```python
from build123d import *

# Parameters (mm, degrees)
F0_R         = 150.3237387913
F0_R_2       = 73.6926609148
F1_DEPTH     = 254
F2_R         = 20.32
F3_R         = 112.9256404591
F3_R_2       = 87.0757104376
F4_DEPTH     = 25.4
F5_R         = 128.6901964601
F6_DEPTH     = 63.5
F7_T4_DEPTH  = 60.7095224794
F7_S5_R      = 128.6901964601
F7_T6_DEPTH  = 32
F7_T10_DEPTH = 60.7095224794
F7_S11_R     = 128.6901964601
F7_T12_DEPTH = 32
F7_T16_DEPTH = 60.7095224794
F7_S17_R     = 128.6901964601
F7_T18_DEPTH = 32
F7_T22_DEPTH = 60.7095224794
F7_S23_R     = 128.6901964601
F7_T24_DEPTH = 32


# Not quite as in the source:
# - a fillet or chamfer that OpenCascade refuses, or shapes differently, is made with other operations: its cross-section is extruded or revolved along the edge and cut away or added


with BuildPart() as f1:
    # F0 (on Front) → F1 (new body)
    with BuildSketch(Plane.XZ):
        Circle(F0_R)
        Circle(F0_R_2, mode=Mode.SUBTRACT)
    extrude(amount=F1_DEPTH)

    # F2
    f2_edges = [f1.edges().sort_by_distance(p)[0] for p in [
        (-150.323739, -254, 0),
    ]]
    fillet(f2_edges, radius=F2_R)

    # F3 (on face) → F4 (join)
    with BuildSketch(Plane(origin=(0, 0, 0), x_dir=(-1, 0, 0), z_dir=(0, 1, 0))):
        Circle(F3_R)
        Circle(F3_R_2, mode=Mode.SUBTRACT)
    extrude(amount=F4_DEPTH)

    # F5 (on Top) → F6 (join, symmetric)
    with BuildSketch(Plane.XY):
        Circle(F5_R)
    extrude(amount=F6_DEPTH, both=True)

    # F7: fillet of radius 5.08 on 4 edges, made by hand


with BuildPart() as f7_tool2:
    # F7_s3 → F7_t4 (new body)
    with BuildSketch(Plane.YZ.offset(-80.6806739807)):
        with BuildLine():
            ThreePointArc((0, -68.58), (1.4878975516, -64.9878975516), (5.08, -63.5))
            Line((5.08, -63.5), (0, -63.5))
            Line((0, -63.5), (0, -68.58))
        make_face()
    extrude(amount=-F7_T4_DEPTH)

    # F7_s5 → F7_t6 (intersect, symmetric)
    with BuildSketch(Plane.XY.offset(-66)):
        Circle(F7_S5_R)
    extrude(amount=F7_T6_DEPTH, both=True, mode=Mode.INTERSECT)


with BuildPart() as f1_1:
    add(f1.part)

    # F7_t1: union F7_tool2
    add(f7_tool2.part)


with BuildPart() as f7_tool8:
    # F7_s9 → F7_t10 (new body)
    with BuildSketch(Plane.YZ.offset(141.3901964601)):
        with BuildLine():
            ThreePointArc((0, -68.58), (1.4878975516, -64.9878975516), (5.08, -63.5))
            Line((5.08, -63.5), (0, -63.5))
            Line((0, -63.5), (0, -68.58))
        make_face()
    extrude(amount=-F7_T10_DEPTH)

    # F7_s11 → F7_t12 (intersect, symmetric)
    with BuildSketch(Plane.XY.offset(-66)):
        Circle(F7_S11_R)
    extrude(amount=F7_T12_DEPTH, both=True, mode=Mode.INTERSECT)


with BuildPart() as f1_2:
    add(f1_1.part)

    # F7_t7: union F7_tool8
    add(f7_tool8.part)


with BuildPart() as f7_tool14:
    # F7_s15 → F7_t16 (new body)
    with BuildSketch(Plane.YZ.offset(-80.6806739807)):
        with BuildLine():
            ThreePointArc((0, 68.58), (1.4878975516, 64.9878975516), (5.08, 63.5))
            Line((5.08, 63.5), (0, 63.5))
            Line((0, 63.5), (0, 68.58))
        make_face()
    extrude(amount=-F7_T16_DEPTH)

    # F7_s17 → F7_t18 (intersect, symmetric)
    with BuildSketch(Plane.XY.offset(66)):
        Circle(F7_S17_R)
    extrude(amount=F7_T18_DEPTH, both=True, mode=Mode.INTERSECT)


with BuildPart() as f1_3:
    add(f1_2.part)

    # F7_t13: union F7_tool14
    add(f7_tool14.part)


with BuildPart() as f7_tool20:
    # F7_s21 → F7_t22 (new body)
    with BuildSketch(Plane.YZ.offset(141.3901964601)):
        with BuildLine():
            ThreePointArc((0, 68.58), (1.4878975516, 64.9878975516), (5.08, 63.5))
            Line((5.08, 63.5), (0, 63.5))
            Line((0, 63.5), (0, 68.58))
        make_face()
    extrude(amount=-F7_T22_DEPTH)

    # F7_s23 → F7_t24 (intersect, symmetric)
    with BuildSketch(Plane.XY.offset(66)):
        Circle(F7_S23_R)
    extrude(amount=F7_T24_DEPTH, both=True, mode=Mode.INTERSECT)


with BuildPart() as f1_4:
    add(f1_3.part)

    # F7_t19: union F7_tool20
    add(f7_tool20.part)


solid = f1_4.part
```
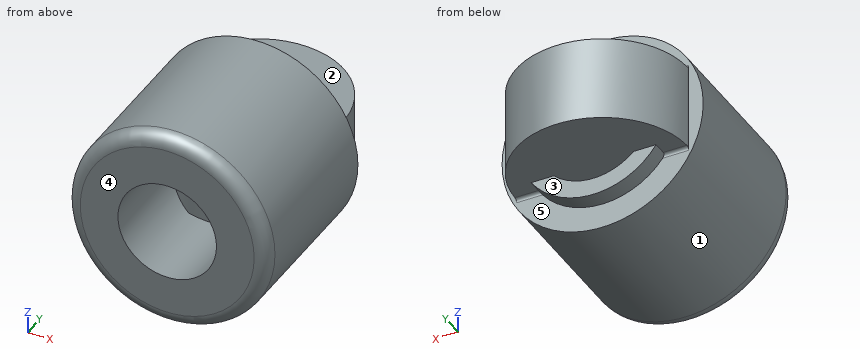
Part model, mm, in its own coordinate system. Face numbers are marked on the shaded views. A direction names the side the tool comes from. Coordinates: 2 decimals unless noted, no trailing zeros. Order: outer loops, then holes, each group sorted by start corner. A loop starts at its lowest first (then second) coordinate and runs counter-clockwise, first axis right, second up. Notation, with made-up numbers: (51, 15) - (102, 15) arc R20 cw to (102, 52) - close; hole circle Ø11 at (76, 57.25). An arc over 180 degrees is marked (long way). Return JSON: item names as keys, results as strings. Group by question number.
Item 1: Which spindle directions (+Z, -Z, +X, -X, +Y, -Y) get a long thin tool onto all of the face, cutting with end or side? Do the marked faces 4 and 5. Say none if no direction does.
Item 2: Cut at C-C (y = -220). List the corners of the cut face in (x, z), plus the area to 3 significant figures.
Item 3: Pin check, flat tips, straight feed: pin 1 (24.5 mm diameter, centred on x = 6, z = -89.5, fed in from +Y); pin 2 (5 mm diameter, centred on y = -47, z = -8, fed in from +X); pin 3 (2 mm diameter, centred on y = 30, z = -24, fed in from +X). Stop position of each tip, or through.
Item 4: Cut at B-B (z = 0). List the corners of the cut face in (x, y), plus the area to 3 significant figures.
Item 5: Drill centre lines: probe 1 along Z at (x, y) = (0, -81.5); probe 2 along Z at (x, y) = (0, -140); probe 3 along Z at (x, y) = (11.5, 11). Where is each one in solid material? Low to high. Write a range as from..to.
Item 6: Cut at A-A (x = 0). List the corners of the cut face in (y, z).
Item 7: Pull direction X, two halves, no side cores. Call the marked faces 1, 2 and 3: pulls with the +X half, pulls with the -X half, needs draft (parallel to the pull), parting line crosses it, or undercut.
Check values:
{
 "1": {"face 4": "+Z, -Z, +X, -X, -Y", "face 5": "+Y"},
 "2": {"outline": "circle Ø300.65 at (0, 0); hole circle Ø147.39 at (0, 0)", "area": "53,900 mm2"},
 "3": {"pin 1": "stops at y = 25.4", "pin 2": "stops at x = 150.22", "pin 3": "stops at x = 125.38"},
 "4": {"outline": "(-150.32, -233.68) arc R20.32 ccw to (-130, -254) - (-73.69, -254) - (-73.69, -105.5) arc R128.69 ccw to (73.69, -105.5) - (73.69, -254) - (130, -254) arc R20.32 ccw to (150.32, -233.68) - (150.32, 0) - (128.69, 0) arc R128.69 ccw to (-128.69, 0) - (-150.32, 0) - close", "area": "82,600 mm2"},
 "5": {"probe 1": "z = -150.32..-73.69, -63.5..63.5, 73.69..150.32", "probe 2": "z = -150.32..-73.69, 73.69..150.32", "probe 3": "z = -112.34..-86.31, -63.5..63.5, 86.31..112.34"},
 "6": {"outline": "(-254, -130) arc R20.32 ccw to (-233.68, -150.32) - (0, -150.32) - (0, -112.93) - (25.4, -112.93) - (25.4, -87.08) - (0, -87.08) - (0, -73.69) - (-254, -73.69) - close; (-254, 73.69) - (0, 73.69) - (0, 87.08) - (25.4, 87.08) - (25.4, 112.93) - (0, 112.93) - (0, 150.32) - (-233.68, 150.32) arc R20.32 ccw to (-254, 130) - close; (-128.69, -63.5) - (128.69, -63.5) - (128.69, 63.5) - (-128.69, 63.5) - close"},
 "7": {"face 1": "parting line crosses it", "face 2": "undercut", "face 3": "needs draft"}
}
